from build123d import *

# Parameters (mm, degrees)
CROQUIS1_W                   = 80
CROQUIS1_H                   = 80
SALIENTE_EXTRUIR1_DEPTH      = 160
CROQUIS2_W                   = 10
CROQUIS2_H                   = 80
CORTAR_EXTRUIR1_DEPTH        = 80
CROQUIS3_W                   = 20
CROQUIS3_H                   = 80
CORTAR_EXTRUIR2_DEPTH        = 80
CROQUIS4_R                   = 20
CORTAR_EXTRUIR3_DEPTH        = 80
CROQUIS5_R                   = 25
SALIENTE_EXTRUIR2_DEPTH      = 30
SALIENTE_EXTRUIR2_DEPTH_BACK = 110


with BuildPart() as part:
    # Croquis1 → Saliente-Extruir1 (new body)
    with BuildSketch(Plane(origin=(0, 0, 0), x_dir=(1, 0, 0), z_dir=(0, 1, 0))):
        with Locations((40, -40)):
            Rectangle(CROQUIS1_W, CROQUIS1_H)
    extrude(amount=SALIENTE_EXTRUIR1_DEPTH)

    # Croquis2 → Cortar-Extruir1 (cut)
    with BuildSketch(Plane(origin=(0, 160, 0), x_dir=(1, 0, 0), z_dir=(0, 1, 0))):
        with Locations((5, -40)):
            Rectangle(CROQUIS2_W, CROQUIS2_H)
        with Locations((75, -40)):
            Rectangle(CROQUIS2_W, CROQUIS2_H)
    extrude(amount=-CORTAR_EXTRUIR1_DEPTH, mode=Mode.SUBTRACT)

    # Croquis3 → Cortar-Extruir2 (cut)
    with BuildSketch(Plane(origin=(0, 160, 0), x_dir=(1, 0, 0), z_dir=(0, 1, 0))):
        with Locations((40, -40)):
            Rectangle(CROQUIS3_W, CROQUIS3_H)
    extrude(amount=-CORTAR_EXTRUIR2_DEPTH, mode=Mode.SUBTRACT)

    # Croquis4 → Cortar-Extruir3 (cut)
    with BuildSketch(Plane(origin=(70, 0, 0), x_dir=(0, 0, -1), z_dir=(1, 0, 0))):
        with BuildLine():
            Line((-80, 160), (-80, 120))
            ThreePointArc((-80, 120), (-68.284271247, 148.284271247), (-40, 160))
            Line((-40, 160), (-80, 160))
        make_face()
        with BuildLine():
            Line((0, 160), (-40, 160))
            ThreePointArc((-40, 160), (-11.715728753, 148.284271247), (0, 120))
            Line((0, 120), (0, 160))
        make_face()
        with Locations((-40, 120)):
            Circle(CROQUIS4_R)
    extrude(amount=-CORTAR_EXTRUIR3_DEPTH, mode=Mode.SUBTRACT)

    # Croquis5 → Saliente-Extruir2 (add, two sides)
    with BuildSketch(Plane(origin=(0, 0, 0), x_dir=(-1, 0, 0), z_dir=(0, 0, -1))) as saliente_extruir2_sk:
        with Locations((-40, 35)):
            Circle(CROQUIS5_R)
    extrude(amount=SALIENTE_EXTRUIR2_DEPTH)
    extrude(saliente_extruir2_sk.sketch, amount=-SALIENTE_EXTRUIR2_DEPTH_BACK)


solid = part.part
Check sheet for the modelled part. Datum: model origin and axes. Units: mm. A direction names the side the tool comes from. Round coordinates to 2 decimals unless told otherwise and drop trailing zeros. Loops run counter-clockwise (first coordinate to the right, second up) from the corner with the lowest first, then second, coordinate; pieces in that order, holes last.
1. Sectioned sample at B-B on x = 24.5. Record the boundary of the cut face in (y, z).
2. Mould release check, pull along X, two halves, no side actions. Record for faces 5 (the flat face through (39, 0, 39)), 6 (the flat face through (10, 94, 41)), 7 (the flat face through (40, 80, 39)): released by +X, released by -X, zero draft, split by the parting line, or undercut.
3. Set-up check for faces 1 (the flat face through (30, 94, 41)), 2 (the flat face through (5, 80, 39)), 3 (the flat face through (70, 94, 41)), 4 (the cylindrical face through (60, 20, 95)): record each of +Z, -Z, +X, -X, +Y, -Y from which the full face is reachable in a straight line by a thin tool's end or side.
4. Gauge pin test, flat ends, axial feed: pin 1 Ø12 at (x, y) = (30, 130.5) entering from -Z; pin 2 Ø3 at (x, z) = (3.5, 39) entering from +Y; pin 3 Ø8 at (y, z) = (58, 13) entering from -X; pin 4 Ø4 at (y, z) = (138.5, 73.5) entering from +X. Record the tip position at first contact, or that the pin passes through.
5. Sectioned sample at C-C on y = 147. Record the boundary of the cut face in (x, z), and give its area (3 significant figures).
6. Sectioned sample at D-D on x = 40. Record the boundary of the cut face in (y, z).
7. Scan lines: probe 1 along X at (y, z) = (84, 52.5); probe 2 along Y at (x, z) = (24.75, 40); probe 3 along Z at (x, y) = (64.5, 53.5). Record each from-to range of solid material in increasing order.
8. Sectioned sample at A-A on y = 113. Record the boundary of the cut face in (x, z) (3 decimals).
Recorded:
1. outline: (0, 0) - (15.38, 0) - (15.38, -30) - (54.62, -30) - (54.62, 0) - (120, 0) arc R40 ccw to (120, 80) - (54.62, 80) - (54.62, 110) - (15.38, 110) - (15.38, 80) - (0, 80) - close; hole circle Ø40 at (120, 40)
2. face 5: zero draft
2. face 6: released by -X
2. face 7: undercut
3. face 1: +Z, -Z, +Y
3. face 2: +Z, -Z, -X, +Y
3. face 3: +Z, -Z, +X, +Y
3. face 4: +Z
4. pin 1: stops at z = 0.25
4. pin 2: stops at y = 80
4. pin 3: stops at x = 0
4. pin 4: stops at x = 70
5. outline: (10, 10.49) - (30, 10.49) - (30, 69.51) - (10, 69.51) - close; (50, 10.49) - (70, 10.49) - (70, 69.51) - (50, 69.51) - close
5. area: 2,360 mm2
6. outline: (0, 0) - (10, 0) - (10, -30) - (60, -30) - (60, 0) - (80, 0) - (80, 80) - (60, 80) - (60, 110) - (10, 110) - (10, 80) - (0, 80) - close
7. probe 1: x = 10 to 30, 50 to 70
7. probe 2: y = 0 to 100, 140 to 160
7. probe 3: z = 0 to 80
8. outline: (10, 0) - (30, 0) - (30, 21.265) - (10, 21.265) - close; (10, 58.735) - (30, 58.735) - (30, 80) - (10, 80) - close; (50, 0) - (70, 0) - (70, 21.265) - (50, 21.265) - close; (50, 58.735) - (70, 58.735) - (70, 80) - (50, 80) - close
